Check sheet for the drawn part. Datum: minimum x, y, z corner. Units: mm. A direction names the side the tool comes from. Round coordinates to 2 decimals unless told otherwise and drop trailing zeros. Write each loop counter-clockwise with the first axis right and the second up, starting at its lowest first coordinate (ties: lowest second). Pieces come first, ordered by that corner, then holes. Notation, with made-up numbers: (33.5, 55) - (40.5, 55) arc R19 cw to (40.5, 91) - close; hole circle Ø11 at (-36.5, -39.75). An arc over 180 degrees is marked (long way). Answer as a JSON object with one key per item and string values.
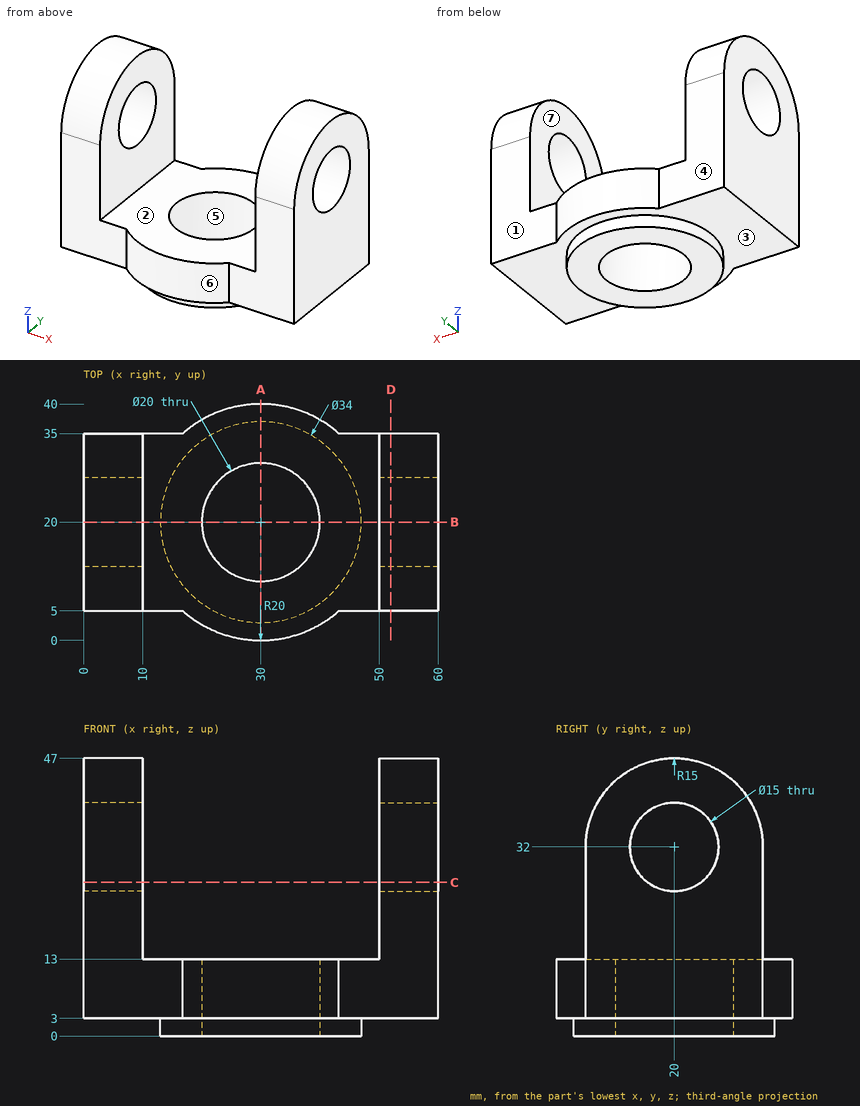
1. Material ranges on probe 1 along X at (y, z) = (25, 15.5); probe 2 along Z at (x, y) = (52.75, 20); probe 3 along Y at (x, z) = (30, 4.25), recorded low to high. Write a range as from..to.
Completed:
{"probe 1": "x = 0..10, 50..60", "probe 2": "z = 3..24.5, 39.5..47", "probe 3": "y = 0..10, 30..40"}
2. Cross-section at C-C (z = 26). Record the boundary of the cut face in (x, y).
Completed:
{"outline": "(0, 5) - (10, 5) - (10, 15.5) - (0, 15.5) - close; (0, 24.5) - (10, 24.5) - (10, 35) - (0, 35) - close; (50, 5) - (60, 5) - (60, 15.5) - (50, 15.5) - close; (50, 24.5) - (60, 24.5) - (60, 35) - (50, 35) - close"}
3. Cross-section at A-A (x = 30). Record the boundary of the cut face in (y, z).
Completed:
{"outline": "(0, 3) - (3, 3) - (3, 0) - (10, 0) - (10, 13) - (0, 13) - close; (30, 0) - (37, 0) - (37, 3) - (40, 3) - (40, 13) - (30, 13) - close"}
4. Mould release check, pull along Y, two halves, no side actions. Record for the marked faces 5, 6 and 7: released by +Y, released by -Y, zero draft, split by the parting line, or undercut.
Completed:
{"face 5": "undercut", "face 6": "released by -Y", "face 7": "zero draft"}
5. Access from +Z, -Z, +X, -X, +Y, -Y to the whole of each face (thin tool, end or side, straight path). Record for the marked faces 1, 2, 3 and 4.
Completed:
{"face 1": "+Z, -Z, +X, +Y", "face 2": "+Z, +Y, -Y", "face 3": "-Z", "face 4": "+Z, -Z, -X, +Y"}
6. Go/stop test with flat-tipped pins: pin 1 (12 mm diameter, centred on x = 22.5, z = 11.5, fed in from +Y); pin 2 (12 mm diameter, centred on x = 23.5, y = 22, fed in from -Z); pin 3 (3 mm diameter, centred on x = 9, y = 24, fed in from +Z); pin 4 (2 mm diameter, centred on x = 7.5, z = 25.5, fed in from -Y). Record where each tip stops, or that it passes through.
Completed:
{"pin 1": "stops at y = 39.94", "pin 2": "stops at z = 0", "pin 3": "stops at z = 46.79", "pin 4": "stops at y = 5"}
7. Cross-section at D-D (x = 52). Record the boundary of the cut face in (y, z), plus the area to 3 significant figures.
Completed:
{"outline": "(5, 3) - (35, 3) - (35, 32) arc R15 ccw to (5, 32) - close; hole circle Ø15 at (20, 32)", "area": "1,050 mm^2"}
8. Cross-section at B-B (y = 20). Record the boundary of the cut face in (x, z), plus the area to 3 significant figures.
Completed:
{"outline": "(0, 3) - (13, 3) - (13, 0) - (20, 0) - (20, 13) - (10, 13) - (10, 24.5) - (0, 24.5) - close; (0, 39.5) - (10, 39.5) - (10, 47) - (0, 47) - close; (40, 0) - (47, 0) - (47, 3) - (60, 3) - (60, 24.5) - (50, 24.5) - (50, 13) - (40, 13) - close; (50, 39.5) - (60, 39.5) - (60, 47) - (50, 47) - close", "area": "822 mm^2"}
